Build history of the part. All positions in model axes, mm. Face numbers are marked on the shaded views. A direction names the side the tool comes from. Give positions to 0.01 mm unless a question says otherwise; leave off trailing zeros. Order: outer loops, then holes, each group sorted by start corner. A loop starts at its lowest first (then second) coordinate and runs counter-clockwise, first axis right, second up. Notation, with made-up numbers: M -30.5,16 L 12.5,16 A16 cw 12.5,40 Z; hole C 60.5,33 d2. An arc over 180 degrees is marked long. One line per item, written item: value.
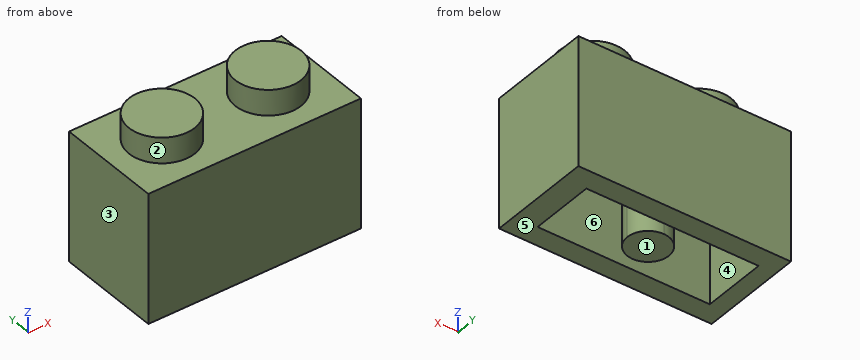
from build123d import *

# Parameters (mm, degrees)
F0_W     = 15.8
F0_H     = 9.6
F1_DEPTH = 7.8
F2_R     = 2.45
F3_DEPTH = 1.9
F5_DEPTH = 8.3
F6_DEPTH = 2


with BuildPart() as f1:
    # F0 (on Front) → F1 (new body)
    with BuildSketch(Plane.XZ):
        with Locations((-46.6530766249, -29.9555875778)):
            Rectangle(F0_W, F0_H)
    extrude(amount=F1_DEPTH)

    # F2 (on face) → F3 (join)
    with BuildSketch(Plane.XY.offset(-25.1555875778)):
        with Locations((-50.6030766249, -3.9)):
            Circle(F2_R)
        with Locations((-42.7030766249, -3.9)):
            Circle(F2_R)
    extrude(amount=F3_DEPTH)

    # F4 (on face) → F5 (cut)
    with BuildSketch(Plane(origin=(0, 0, -34.7555875778), x_dir=(1, 0, 0), z_dir=(0, 0, -1))):
        with BuildLine():
            Line((-53.2821939588, 6.3), (-53.2821939588, 1.5))
            Line((-53.2821939588, 1.5), (-46.8821939588, 1.5))
            Line((-46.8821939588, 1.5), (-46.8821939588, 1.925))
            Line((-46.8821939588, 1.925), (-46.8821939588, 2.35))
            ThreePointArc((-46.8821939588, 2.35), (-48.4321435514, 3.8874995935), (-46.9071939588, 5.449798374))
            Line((-46.9071939588, 5.449798374), (-46.9071939588, 6.3))
            Line((-46.9071939588, 6.3), (-53.2821939588, 6.3))
        make_face()
        with BuildLine():
            Line((-46.8821939588, 1.925), (-46.8821939588, 1.5))
            Line((-46.8821939588, 1.5), (-40.4821939588, 1.5))
            Line((-40.4821939588, 1.5), (-40.4821939588, 6.3))
            Line((-40.4821939588, 6.3), (-46.8571939588, 6.3))
            Line((-46.8571939588, 6.3), (-46.8571939588, 5.449798374))
            ThreePointArc((-46.8571939588, 5.449798374), (-45.7773749691, 4.9871407453), (-45.3321939588, 3.9))
            ThreePointArc((-45.3321939588, 3.9), (-45.7861784479, 2.8039844892), (-46.8821939588, 2.35))
            Line((-46.8821939588, 2.35), (-46.8821939588, 1.925))
        make_face()
    extrude(amount=-F5_DEPTH, mode=Mode.SUBTRACT)

    # F4 (on face) → F6 (cut)
    with BuildSketch(Plane(origin=(0, 0, -34.7555875778), x_dir=(1, 0, 0), z_dir=(0, 0, -1))):
        with BuildLine():
            Line((-46.8571939588, 6.3), (-46.9071939588, 6.3))
            Line((-46.9071939588, 6.3), (-46.9071939588, 5.449798374))
            ThreePointArc((-46.9071939588, 5.449798374), (-46.8821939588, 5.45), (-46.8571939588, 5.449798374))
            Line((-46.8571939588, 5.449798374), (-46.8571939588, 6.3))
        make_face()
    extrude(amount=-F6_DEPTH, mode=Mode.SUBTRACT)


solid = f1.part
1) Saw through at D-D, the plane x = -48.75. Write the cut outline in (y, z).
Check values:
outline: M -7.8,-34.76 L -6.3,-34.76 L -6.3,-26.46 L -1.5,-26.46 L -1.5,-34.76 L 0,-34.76 L 0,-25.16 L -2.3,-25.16 L -2.3,-23.26 L -5.5,-23.26 L -5.5,-25.16 L -7.8,-25.16 Z
2) Saw through at A-A, the plane z = -32. Write the cut outline in (x, y), then the cut area to 3 significant figures.
Check values:
outline: M -54.55,-7.8 L -38.75,-7.8 L -38.75,0 L -54.55,0 Z; hole M -53.28,-6.3 L -46.91,-6.3 L -46.91,-5.45 A1.55 cw long -46.86,-5.45 L -46.86,-6.3 L -40.48,-6.3 L -40.48,-1.5 L -53.28,-1.5 Z
area: 69.4 mm^2
3) Tool access for the marked faces 1 and 2: list every direction of +Z, -Z, +X, -X, +Y, -Y with a clear straight run to the whole face (end or side of a thin tool).
Check values:
face 1: -Z, +X, -X, +Y, -Y
face 2: +Z
4) Mould opens along X. For the marked faces 3, 4, 5 and 6 say: released by +X, released by -X, zero draft, split by the parting line, or undercut.
Check values:
face 3: released by -X
face 4: undercut
face 5: zero draft
face 6: undercut
5) Saw through at C-C, the plane y = -4.5. Write the cut outline in (x, z).
Check values:
outline: M -54.55,-34.76 L -53.28,-34.76 L -53.28,-26.46 L -48.31,-26.46 L -48.31,-34.76 L -45.45,-34.76 L -45.45,-26.46 L -40.48,-26.46 L -40.48,-34.76 L -38.75,-34.76 L -38.75,-25.16 L -40.33,-25.16 L -40.33,-23.26 L -45.08,-23.26 L -45.08,-25.16 L -48.23,-25.16 L -48.23,-23.26 L -52.98,-23.26 L -52.98,-25.16 L -54.55,-25.16 Z
6) Saw through at B-B, the plane x = -52.25. Write the cut outline in (y, z).
Check values:
outline: M -7.8,-34.76 L -6.3,-34.76 L -6.3,-26.46 L -1.5,-26.46 L -1.5,-34.76 L 0,-34.76 L 0,-25.16 L -2.09,-25.16 L -2.09,-23.26 L -5.71,-23.26 L -5.71,-25.16 L -7.8,-25.16 Z
7) Pin check, flat tip, straight feed: pin 1 (6 mm diameter, centred on x = -49, z = -24.5, fed in from -Y). Stop position of the tip, or through.
Check values:
pin 1: y = -7.8
8) Drill centre lines: probe 1 along X at (y, z) = (-4, -30); probe 2 along Y at (x, z) = (-50.75, -32); probe 3 along X at (y, z) = (-4.25, -32.5). Where is each one in solid material? Low to high. Write a range as from..to.
Check values:
probe 1: -54.55..-53.28, -48.43..-45.34, -40.48..-38.75
probe 2: -7.8..-6.3, -1.5..0
probe 3: -54.55..-53.28, -48.39..-45.37, -40.48..-38.75
